from build123d import *

# Parameters (mm, degrees)
BOSS_EXTRUDE3_DEPTH      = 4.826
BOSS_EXTRUDE3_DEPTH_BACK = 4.826
CUT_EXTRUDE1_DEPTH       = 4.572


with BuildPart() as part:
    # Sketch1 → Boss-Extrude3 (new body, two sides)
    with BuildSketch(Plane(origin=(0, 0, 0), x_dir=(1, 0, 0), z_dir=(0, 1, 0))) as boss_extrude3_sk:
        with BuildLine():
            Line((17.147972, 0.440697), (8.627907, 0.440697))
            ThreePointArc((8.627907, 0.440697), (8.825999, -0.18062), (8.892972, -0.829303))
            ThreePointArc((8.892972, -0.829303), (8.770347, -1.703161), (8.411946, -2.509519))
            Line((8.411946, -2.509519), (15.174656, -2.509519))
            ThreePointArc((15.174656, -2.509519), (15.674194, -0.70859), (17.147972, 0.440697))
        make_face()
        with BuildLine():
            ThreePointArc((21.13129, -2.365409), (19.867474, 0.070831), (17.147972, 0.440697))
            ThreePointArc((17.147972, 0.440697), (15.674194, -0.70859), (15.174656, -2.509519))
            ThreePointArc((15.174656, -2.509519), (18.223306, -5.344597), (21.13129, -2.365409))
        make_face()
        with BuildLine():
            ThreePointArc((8.627907, 0.440697), (7.456991, 1.827093), (5.717972, 2.345697))
            Line((5.717972, 2.345697), (5.717972, 0.186697))
            ThreePointArc((5.717972, 0.186697), (6.436392, -0.110882), (6.733972, -0.829303))
            ThreePointArc((6.733972, -0.829303), (6.436392, -1.547723), (5.717972, -1.845303))
            Line((5.717972, -1.845303), (5.717972, -4.004303))
            ThreePointArc((5.717972, -4.004303), (7.258416, -3.605569), (8.411946, -2.509519))
            ThreePointArc((8.411946, -2.509519), (8.770347, -1.703161), (8.892972, -0.829303))
            ThreePointArc((8.892972, -0.829303), (8.825999, -0.18062), (8.627907, 0.440697))
        make_face()
        with BuildLine():
            Line((5.717972, 0.186697), (5.717972, 2.345697))
            ThreePointArc((5.717972, 2.345697), (2.542972, -0.829303), (5.717972, -4.004303))
            Line((5.717972, -4.004303), (5.717972, -1.845303))
            ThreePointArc((5.717972, -1.845303), (4.701972, -0.829303), (5.717972, 0.186697))
        make_face()
        with BuildLine():
            Line((5.717972, 2.345697), (5.717972, 4.530275))
            ThreePointArc((5.717972, 4.530275), (0.358393, -0.829303), (5.717972, -6.188881))
            Line((5.717972, -6.188881), (5.717972, -4.004303))
            ThreePointArc((5.717972, -4.004303), (2.542972, -0.829303), (5.717972, 2.345697))
        make_face()
    extrude(amount=BOSS_EXTRUDE3_DEPTH)
    extrude(boss_extrude3_sk.sketch, amount=-BOSS_EXTRUDE3_DEPTH_BACK)

    # Sketch4 → Cut-Extrude1 (cut)
    with BuildSketch(Plane(origin=(0, 4.826, 0), x_dir=(1, 0, 0), z_dir=(0, 1, 0))):
        with BuildLine():
            ThreePointArc((8.892972, -0.829303), (8.770347, -1.703161), (8.411946, -2.509519))
            Line((8.411946, -2.509519), (14.979502, -2.509519))
            ThreePointArc((14.979502, -2.509519), (15.394758, -0.789818), (16.665836, 0.440697))
            Line((16.665836, 0.440697), (8.627907, 0.440697))
            ThreePointArc((8.627907, 0.440697), (8.825999, -0.18062), (8.892972, -0.829303))
        make_face()
    extrude(amount=-CUT_EXTRUDE1_DEPTH, mode=Mode.SUBTRACT)


solid = part.part
Verification items for the finished model (mm, model axes). A direction names the side the tool comes from. Coordinates: 2 decimals unless noted, no trailing zeros. Order: outer loops, then holes, each group sorted by start corner. A loop starts at its lowest first (then second) coordinate and runs counter-clockwise, first axis right, second up. Notation, with made-up numbers: M -20.5,-15.75 L 21.5,-15.75 A22 cw 21.5,19.25 Z; hole C -29,-22.5 d3. An arc over 180 degrees is marked long. One line per item, written item: value. Start each with the question number.
Item 1: Access from +Z, -Z, +X, -X, +Y, -Y to the whole of each face (thin tool, end or side, straight path). Record for faces 1 (the flat face through (18, 4.826, 2)), 2 (the flat face through (5.718, 0, 5)), 3 (the flat face through (11, -4.826, 1)), 4 (the flat face through (13, -2, -0.441)), 5 (the flat face through (5.718, 0, -3)).
Item 2: Sectioned sample at B-B (z = 3.75). Enter the section's corners in (x, y).
Item 3: Sectioned sample at D-D (x = 14). Enter the section's corners in (y, z).
Item 4: Sectioned sample at C-C (y = 3.75). Count the separate pieces of the cut face and the enclosed holes in it, then the cut area to 3 significant figures.
Item 5: Scan lines: probe 1 along Z at (x, y) = (5.75, 1.5); probe 2 along Z at (x, y) = (18, -4.25); probe 3 along Y at (x, z) = (15.5, 0.5). Record each from-to range of solid material in increasing order.
Item 6: Gauge pin test, flat ends, axial feed: pin 1 (4 mm diameter, centred on x = 12, z = -1.5, fed in from +Y); pin 2 (1.1 mm diameter, centred on y = 0, z = 5, fed in from +X); pin 3 (1.5 mm diameter, centred on x = 11, y = -2, fed in from +Z). Record the tip position at first contact, or that the pin passes through.
Item 7: Mould release check, pull along X, two halves, no side actions. Record for faces 6 (the cylindrical face through (0.36, 0.07, 0.71)), 7 (the flat face through (4, 4.826, 1)), 8 (the flat face through (12, -2, 2.51)): released by +X, released by -X, zero draft, split by the parting line, or undercut.
Conclusion:
1. face 1: +Z, -Z, +X, -X, +Y
1. face 2: +Z, +Y, -Y
1. face 3: +Z, -Z, +X, -X, -Y
1. face 4: -Z, +Y, -Y
1. face 5: -Z, +X, +Y, -Y
2. outline: M 1.22,-4.83 L 6.96,-4.83 L 6.96,4.83 L 1.22,4.83 Z; M 15.51,-4.83 L 20.79,-4.83 L 20.79,4.83 L 15.51,4.83 Z
3. outline: M -4.83,-0.44 L 0.25,-0.44 L 0.25,2.51 L -4.83,2.51 Z
4. separate pieces: 2
4. enclosed holes: 1
4. area: 86.3 mm^2
5. probe 1: z = -2.35 to -0.19, 1.84 to 4
5. probe 2: z = -0.61 to 5.34
5. probe 3: y = -4.83 to 0.25
6. pin 1: stops at y = 0.25
6. pin 2: stops at x = 20.28
6. pin 3: stops at z = 2.51
7. face 6: released by -X
7. face 7: zero draft
7. face 8: undercut
